Geometry check sheet. Reference: the model listing, model coordinates, mm. A direction names the side the tool comes from. Round coordinates to 2 decimals unless told otherwise and drop trailing zeros. Write each loop counter-clockwise with the first axis right and the second up, starting at its lowest first coordinate (ties: lowest second). Pieces come first, ordered by that corner, then holes. Notation, with made-up numbers: M 89,-8 L 146,-8 A12 ccw 146,13 Z; hole C -25,4 d3. An arc over 180 degrees is marked long. One line per item, written item: value. Start each with the question number.
1. Section check D-D (x = 125). Record the boundary of the cut face in (y, z).
2. Depth check by flat-ended pin: P1, Ø3, axis at x = 79.5, z = 564.5, coming from the +Y side. Enter the tip coordinate at first touch or a pass-through.
3. Access from +Z, -Z, +X, -X, +Y, -Y to the whole of each face (thin tool, end or side, straight path). Record for faces 1 (the flat face through (127, 123, 15)), 2 (the flat face through (123, -15, 507)).
4. Section check A-A (y = 200). Record the boundary of the cut face in (x, z).
5. Scan lines: probe 1 along X at (y, z) = (200, 4); probe 2 along X at (y, z) = (35, 11); probe 3 along Y at (x, z) = (125, 8). Record each from-to range of solid material in increasing order. Write a range as [from, to].
6. Section check B-B (y = 35). Record the boundary of the cut face in (x, z).
7. Release check for a two-part mould opening along Z. For faces 3 (the cylindrical face through (5.703, -7.605, 993.986)), 4 (the cylindrical face through (184.68, 190.54, 7.4)), 5 (the cylindrical face through (123.698, -7.605, 492.915)), 6 (the cylindrical face through (123.698, -7.605, 727.915)) record: pulls with the +Z half, pulls with the -Z half, needs draft (parallel to the pull), parting line crosses it, or undercut.
8. Section check C-C (z = 718). Record the boundary of the cut face in (x, y).
from build123d import *

# Parameters (mm, degrees)
F0_W      = 250
F0_H      = 1000
F1_DEPTH  = 15
F2_R      = 20
F3_R      = 20
F4_W      = 250
F4_H      = 15
F5_DEPTH  = 250
F7_DEPTH  = 15
F9_DEPTH  = 15
F10_R     = 14
F11_DEPTH = 15
F12_R     = 10
F13_DEPTH = 265.001


with BuildPart() as f1:
    # F0 (on Front) → F1 (new body)
    with BuildSketch(Plane.XZ):
        with Locations((125, 500)):
            Rectangle(F0_W, F0_H)
    extrude(amount=F1_DEPTH)

    # F2
    f2_edges = [f1.edges().sort_by_distance(p)[0] for p in [
        (0, -7.5, 1000),
    ]]
    fillet(f2_edges, radius=F2_R)

    # F3
    f3_edges = [f1.edges().sort_by_distance(p)[0] for p in [
        (250, -7.5, 1000),
    ]]
    fillet(f3_edges, radius=F3_R)

    # F4 (on face) → F5 (join)
    with BuildSketch(Plane(origin=(0, 0, 0), x_dir=(-1, 0, 0), z_dir=(0, 1, 0))):
        with Locations((-125, 7.5)):
            Rectangle(F4_W, F4_H)
    extrude(amount=F5_DEPTH)

    # F6 (on face) → F7 (join)
    with BuildSketch(Plane(origin=(0, 0, 0), x_dir=(0, -1, 0), z_dir=(-1, 0, 0))):
        Polygon((0, 315), (-250, 15), (0, 15), align=None)
    extrude(amount=-F7_DEPTH)

    # F8 (on face) → F9 (join)
    with BuildSketch(Plane.YZ.offset(250)):
        Polygon((0, 15), (250, 15), (0, 315), align=None)
    extrude(amount=-F9_DEPTH)

    # F10 (on face) → F11 (cut)
    with BuildSketch(Plane(origin=(0, 0, 0), x_dir=(1, 0, 0), z_dir=(0, 0, -1))):
        with Locations((125, -35)):
            Circle(F10_R)
        with Locations((195, -200)):
            Circle(F10_R)
        with Locations((55, -200)):
            Circle(F10_R)
    extrude(amount=-F11_DEPTH, mode=Mode.SUBTRACT)

    # F12 (on face) → F13 (cut, through all)
    with BuildSketch(Plane.XZ.offset(15)):
        with Locations((125, 718)):
            Circle(F12_R)
        with Locations((125, 483)):
            Circle(F12_R)
    extrude(amount=-F13_DEPTH, mode=Mode.SUBTRACT)


solid = f1.part
Result sheet:
1. outline: M -15,0 L 21,0 L 21,15 L 0,15 L 0,473 L -15,473 Z; M -15,493 L 0,493 L 0,708 L -15,708 Z; M -15,728 L 0,728 L 0,1000 L -15,1000 Z; M 49,0 L 250,0 L 250,15 L 49,15 Z
2. P1: stops at y = 0
3. face 1: +Z, +Y
3. face 2: +Z, -Z, +X, -X, -Y
4. outline: M 0,0 L 41,0 L 41,15 L 15,15 L 15,75 L 0,75 Z; M 69,0 L 181,0 L 181,15 L 69,15 Z; M 209,0 L 250,0 L 250,75 L 235,75 L 235,15 L 209,15 Z
5. probe 1: x = [0, 41], [69, 181], [209, 250]
5. probe 2: x = [0, 111], [139, 250]
5. probe 3: y = [-15, 21], [49, 250]
6. outline: M 0,0 L 111,0 L 111,15 L 15,15 L 15,273 L 0,273 Z; M 139,0 L 250,0 L 250,273 L 235,273 L 235,15 L 139,15 Z
7. face 3: pulls with the +Z half
7. face 4: needs draft
7. face 5: undercut
7. face 6: undercut
8. outline: M 0,-15 L 115,-15 L 115,0 L 0,0 Z; M 135,-15 L 250,-15 L 250,0 L 135,0 Z
